For this review, take the finished solid that the model builds, in its own axes (mm). A direction names the side the tool comes from. Round coordinates to 2 decimals unless told otherwise and drop trailing zeros. Order: outer loops, then holes, each group sorted by start corner. A loop starts at its lowest first (then second) coordinate and runs counter-clockwise, first axis right, second up. Notation, with made-up numbers: M 47.5,4.25 L 67.5,4.25 A12 cw 67.5,21.25 Z; hole C 13.5,59 d2. An arc over 180 degrees is marked long. Put each result on its own line as item: value.
from build123d import *

# Parameters (mm, degrees)
CROQUIS1_R              = 2.5
SALIENTE_EXTRUIR1_DEPTH = 144


with BuildPart() as part:
    # Croquis1 → Saliente-Extruir1 (new body)
    with BuildSketch(Plane.XY):
        with BuildLine():
            Line((-4.6, 10), (-3.1, 8.5))
            Line((-3.1, 8.5), (-3.1, 8.2))
            Line((-3.1, 8.2), (-5.5, 8.2))
            Line((-5.5, 8.2), (-5.5, 6.560660172))
            Line((-5.5, 6.560660172), (-2.84, 3.900660172))
            Line((-2.84, 3.900660172), (0, 3.900660172))
            Line((0, 3.900660172), (2.84, 3.900660172))
            Line((2.84, 3.900660172), (5.5, 6.560660172))
            Line((5.5, 6.560660172), (5.5, 8.2))
            Line((5.5, 8.2), (3.1, 8.2))
            Line((3.1, 8.2), (3.1, 8.5))
            Line((3.1, 8.5), (4.6, 10))
            Line((4.6, 10), (9.25, 10))
            ThreePointArc((9.25, 10), (9.780330086, 9.780330086), (10, 9.25))
            Line((10, 9.25), (10, 4.6))
            Line((10, 4.6), (8.5, 3.1))
            Line((8.5, 3.1), (8.2, 3.1))
            Line((8.2, 3.1), (8.2, 5.5))
            Line((8.2, 5.5), (6.560660172, 5.5))
            Line((6.560660172, 5.5), (3.900660172, 2.84))
            Line((3.900660172, 2.84), (3.900660172, 0))
            Line((3.900660172, 0), (3.900660172, -2.84))
            Line((3.900660172, -2.84), (6.560660172, -5.5))
            Line((6.560660172, -5.5), (8.2, -5.5))
            Line((8.2, -5.5), (8.2, -3.1))
            Line((8.2, -3.1), (8.5, -3.1))
            Line((8.5, -3.1), (10, -4.6))
            Line((10, -4.6), (10, -9.25))
            ThreePointArc((10, -9.25), (9.780330086, -9.780330086), (9.25, -10))
            Line((9.25, -10), (4.6, -10))
            Line((4.6, -10), (3.1, -8.5))
            Line((3.1, -8.5), (3.1, -8.2))
            Line((3.1, -8.2), (5.5, -8.2))
            Line((5.5, -8.2), (5.5, -6.560660172))
            Line((5.5, -6.560660172), (2.84, -3.900660172))
            Line((2.84, -3.900660172), (0, -3.900660172))
            Line((0, -3.900660172), (-2.84, -3.900660172))
            Line((-2.84, -3.900660172), (-5.5, -6.560660172))
            Line((-5.5, -6.560660172), (-5.5, -8.2))
            Line((-5.5, -8.2), (-3.1, -8.2))
            Line((-3.1, -8.2), (-3.1, -8.5))
            Line((-3.1, -8.5), (-4.6, -10))
            Line((-4.6, -10), (-9.25, -10))
            ThreePointArc((-9.25, -10), (-9.780330086, -9.780330086), (-10, -9.25))
            Line((-10, -9.25), (-10, -4.6))
            Line((-10, -4.6), (-8.5, -3.1))
            Line((-8.5, -3.1), (-8.2, -3.1))
            Line((-8.2, -3.1), (-8.2, -5.5))
            Line((-8.2, -5.5), (-6.560660172, -5.5))
            Line((-6.560660172, -5.5), (-3.900660172, -2.84))
            Line((-3.900660172, -2.84), (-3.900660172, 0))
            Line((-3.900660172, 0), (-3.900660172, 2.84))
            Line((-3.900660172, 2.84), (-6.560660172, 5.5))
            Line((-6.560660172, 5.5), (-8.2, 5.5))
            Line((-8.2, 5.5), (-8.2, 3.1))
            Line((-8.2, 3.1), (-8.5, 3.1))
            Line((-8.5, 3.1), (-10, 4.6))
            Line((-10, 4.6), (-10, 9.25))
            ThreePointArc((-10, 9.25), (-9.780330086, 9.780330086), (-9.25, 10))
            Line((-9.25, 10), (-4.6, 10))
        make_face()
        Circle(CROQUIS1_R, mode=Mode.SUBTRACT)
    extrude(amount=SALIENTE_EXTRUIR1_DEPTH)


solid = part.part
(1) Insertion check: pin 1 Ø8 at (x, y) = (1, -5) entering from +Z; pin 2 Ø3 at (x, y) = (0, 0) entering from +Z; pin 3 Ø2 at (x, z) = (-2.5, 77.5) entering from +Y; pin 4 Ø3 at (y, z) = (3, 38) entering from -X. Each pin has a flat end and moves straight along its axis. Give the tip position at first contact, or say it passes through.
A:
pin 1: stops at z = 144
pin 2: passes through
pin 3: stops at y = 8.9
pin 4: stops at x = -9.9
(2) Draft analysis for pull direction X (two halves, no side actions). For faces 4 (the face through (-2, 2, 0)), 5 (the face through (-5.21, 4.15, 70.99)), 6 (the face through (10, -7, 71)), state which applies: released by +X, released by -X, zero draft, split by the parting line, or undercut.
A:
face 4: zero draft
face 5: undercut
face 6: released by +X
(3) For faces 1 (the face through (0, 3.901, 71)), 2 (the face through (-4, -8.2, 71)), 3 (the face through (-10, -7, 71)), list the 3-axis set-ups (+Z, -Z, +X, -X, +Y, -Y) from which the entire face can be reached by the end or side of a thin tool; tool diameter is ignored.
A:
face 1: +Z, -Z, +Y
face 2: +Z, -Z
face 3: +Z, -Z, -X, +Y, -Y
(4) Add section A-A on y = 0. Give the boundary of the cut face in (x, z), then the cut area to 3 significant figures.
A:
outline: M -3.9,0 L -2.5,0 L -2.5,144 L -3.9,144 Z; M 2.5,0 L 3.9,0 L 3.9,144 L 2.5,144 Z
area: 403 mm2
(5) To check wall thickness, follow L1, parallel to Y at x = 0, z = 134.5; L2, parallel to Y at x = 7.25, z = 37.5. State the ranges of each line that lie inside material, in increasing order.
A:
L1: y = -3.9 to -2.5, 2.5 to 3.9
L2: y = -10 to -5.5, 5.5 to 10
